from build123d import *

# Parameters (mm, degrees)
BOSS_EXTRUDE1_DEPTH = 6.35
SKETCH2_R           = 1.524
BOSS_EXTRUDE2_DEPTH = 7.366
DOME1_FACE_RADIUS   = 1.524
DOME1_HEIGHT        = 1.524
DOME2_FACE_RADIUS   = 1.524
DOME2_HEIGHT        = 1.524
BOSS_EXTRUDE3_DEPTH = 4.572
BOSS_EXTRUDE4_DEPTH = 4.572


with BuildPart() as part:
    # Sketch1 → Boss-Extrude1 (new body)
    with BuildSketch(Plane(origin=(0, 0, 0), x_dir=(0, 0, -1), z_dir=(1, 0, 0))):
        with BuildLine():
            Line((-4.318, -9.398), (5.588, -9.398))
            Line((5.588, -9.398), (5.588, 9.398))
            Line((5.588, 9.398), (-4.318, 9.398))
            ThreePointArc((-4.318, 9.398), (-5.216025612, 9.026025612), (-5.588, 8.128))
            Line((-5.588, 8.128), (-5.588, -8.128))
            ThreePointArc((-5.588, -8.128), (-5.216025612, -9.026025612), (-4.318, -9.398))
        make_face()
    extrude(amount=-BOSS_EXTRUDE1_DEPTH)

    # Sketch2 → Boss-Extrude2 (add)
    with BuildSketch(Plane(origin=(0, 0, 0), x_dir=(0, 0, -1), z_dir=(1, 0, 0))):
        with Locations((0.508, -2.794)):
            Circle(SKETCH2_R)
        with Locations((0.508, 3.81)):
            Circle(SKETCH2_R)
    extrude(amount=BOSS_EXTRUDE2_DEPTH)

    # Dome1: a dome of height H over a round flat face of radius A is a cap of a sphere of radius (A * A + H * H) / (2 * H)
    dome1_r = (DOME1_FACE_RADIUS * DOME1_FACE_RADIUS + DOME1_HEIGHT * DOME1_HEIGHT) / (2 * DOME1_HEIGHT)
    dome1_base = Plane((7.366, 3.81, -0.508), z_dir=(1, 0, 0))
    with Locations(dome1_base.offset(DOME1_HEIGHT - dome1_r)):
        dome1_ball = Sphere(dome1_r, mode=Mode.PRIVATE)
    add(split(dome1_ball, bisect_by=dome1_base, keep=Keep.TOP, mode=Mode.PRIVATE))

    # Dome2: a dome of height H over a round flat face of radius A is a cap of a sphere of radius (A * A + H * H) / (2 * H)
    dome2_r = (DOME2_FACE_RADIUS * DOME2_FACE_RADIUS + DOME2_HEIGHT * DOME2_HEIGHT) / (2 * DOME2_HEIGHT)
    dome2_base = Plane((7.366, -2.794, -0.508), z_dir=(1, 0, 0))
    with Locations(dome2_base.offset(DOME2_HEIGHT - dome2_r)):
        dome2_ball = Sphere(dome2_r, mode=Mode.PRIVATE)
    add(split(dome2_ball, bisect_by=dome2_base, keep=Keep.TOP, mode=Mode.PRIVATE))

    # Sketch6 → Boss-Extrude3 (add)
    with BuildSketch(Plane.XY.offset(1.778)):
        with BuildLine():
            Line((-6.35, -3.391509029), (-6.35, -9.68399892))
            ThreePointArc((-6.35, -9.68399892), (-6.935786754, -11.098213246), (-8.35000108, -11.684))
            Line((-8.35000108, -11.684), (-28.448, -11.684))
            Line((-28.448, -11.684), (-31.242, -10.381136403))
            Line((-31.242, -10.381136403), (-31.242, -10.344325173))
            Line((-31.242, -10.344325173), (-28.424812359, -11.6586))
            Line((-28.424812359, -11.6586), (-8.35000108, -11.6586))
            ThreePointArc((-8.35000108, -11.6586), (-6.953747266, -11.080252734), (-6.3754, -9.68399892))
            Line((-6.3754, -9.68399892), (-6.3754, -3.391509029))
            Line((-6.3754, -3.391509029), (-6.35, -3.391509029))
        make_face()
    extrude(amount=-BOSS_EXTRUDE3_DEPTH)

    # Sketch7 → Boss-Extrude4 (add)
    with BuildSketch(Plane.XY.offset(1.778)):
        with BuildLine():
            Line((-6.35, 5.171328303), (-6.35, -0.851509029))
            Line((-6.35, -0.851509029), (-31.14416134, -9.87584574))
            Line((-31.14416134, -9.87584574), (-31.14416134, -9.848815625))
            Line((-31.14416134, -9.848815625), (-6.3754, -0.833723757))
            Line((-6.3754, -0.833723757), (-6.3754, 5.171328303))
            ThreePointArc((-6.3754, 5.171328303), (-6.3627, 5.184028303), (-6.35, 5.171328303))
        make_face()
    extrude(amount=-BOSS_EXTRUDE4_DEPTH)


solid = part.part
The listing builds one solid part. Answer for the finished solid, in the listing's coordinates (mm). A direction names the side the tool comes from. Give positions to 0.01 mm unless a question says otherwise; leave off trailing zeros. Loops run counter-clockwise (first coordinate to the right, second up) from the corner with the lowest first, then second, coordinate; pieces in that order, holes last. Notation, with made-up numbers: (55, 31) - (109, 31) arc R33 ccw to (109, 59) - close; hole circle Ø7 at (30.25, 61.25). An arc over 180 degrees is marked (long way). Answer as a JSON object with one key per item and string values.
1. Find the intervals of material crossed by L1, parallel to X at y = 3.25, z = 3; L2, parallel to Y at x = -2, z = -2; L3, parallel to Z at x = 2.5, y = -1.5, in increasing order. Write a range as [from, to].
Determined:
{"L1": "[-6.35, 0]", "L2": "[-9.4, 9.4]", "L3": "[-1.31, 0.3]"}
2. Flat-ended cylindrical pins translate along their axes: pin 1 Ø2.5 at (x, z) = (-17.5, -1) entering from +Y; pin 2 Ø3.5 at (y, z) = (3, -2.5) entering from -X; pin 3 Ø1.5 at (y, z) = (-1.5, -0.5) entering from +X. Find the tip coordinate at first contact, or state that the pin passes through.
Determined:
{"pin 1": "y = -4.43", "pin 2": "x = -6.38", "pin 3": "x = 8.79"}
3. For a pull along Y with two mould halves and no side action, classify faces 4 (the cylindrical face through (-3.131, 9.036, 5.206)), 5 (the cylindrical face through (4, -3, 1)), 6 (the cylindrical face through (-3.131, -9.016, 5.226)) as pulls with the +Y half, pulls with the -Y half, needs draft (parallel to the pull), parting line crosses it, or undercut.
Determined:
{"face 4": "pulls with the +Y half", "face 5": "undercut", "face 6": "pulls with the -Y half"}
4. A cutting plane is placed at D-D (x = -2). Write down the section's boundary in (y, z).
Determined:
{"outline": "(-9.4, -5.59) - (9.4, -5.59) - (9.4, 4.32) arc R1.27 ccw to (8.13, 5.59) - (-8.13, 5.59) arc R1.27 ccw to (-9.4, 4.32) - close"}
5. For faces 1 (the flat face through (-3, 0, -5.588)), 2 (the cylindrical face through (3.63, 5.32, -0.31)), 3 (the flat face through (-3, -9.398, -1)), determine the directions among +Z, -Z, +X, -X, +Y, -Y from which every point of the face is accessible in a straight line to the end or side of a thin tool.
Determined:
{"face 1": "-Z, +X, -X, +Y, -Y", "face 2": "+X", "face 3": "+Z, -Z, +X, -Y"}
